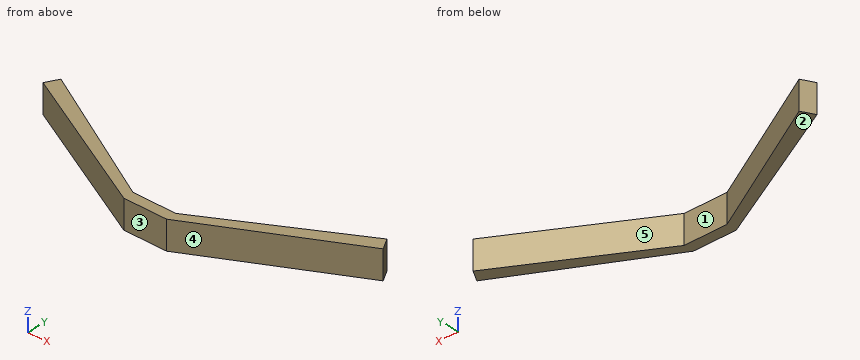
from build123d import *

# Parameters (mm, degrees)
F0_W     = 7.947458
F0_H     = 1.932221
F1_DEPTH = 5.334


with BuildPart() as f1:
    # F0 (on Top) → F1 (new body)
    with BuildSketch(Plane.XY):
        Polygon((18.552113, 1.932221), (18.552113, 0), (45.986039, 14.360375), (44.759143, 16.558673), align=None)
        Polygon((-17.014322, 14.249988), (10.604655, 0), (10.604655, 1.932221), (-15.732167, 16.558673), align=None)
        with Locations((14.578384, 0.96611)):
            Rectangle(F0_W, F0_H)
    extrude(amount=F1_DEPTH)


solid = f1.part
Read the model definition and answer for the solid it produces. Units are mm, in the model's axes. Face numbers are marked on the shaded views. A direction names the side the tool comes from. Round coordinates to 2 decimals unless told otherwise and drop trailing zeros. Write each loop counter-clockwise with the first axis right and the second up, starting at its lowest first coordinate (ties: lowest second). Pieces come first, ordered by that corner, then holes. Notation, with made-up numbers: (88.5, 75.25) - (112.5, 75.25) arc R14 ccw to (112.5, 98.25) - close; hole circle Ø1 at (9.5, 28.25). An arc over 180 degrees is marked (long way). Use a Markdown table: item, result.
(1) Straight lines are drawn through the part: line 1 along X through (y, z) = (2, 2.3); line 2 along X through (y, z) = (11.25, 2.85); line 3 along Y through (x, z) = (14, 4.15). For each, find the intervals that lie inside material, in ascending order. Write a range as [from, to].
Reported:
| item | result |
|---|---|
| line 1 | [6.73, 10.48], [18.67, 22.37] |
| line 2 | [-11.2, -6.17], [35.25, 40.04] |
| line 3 | [0, 1.93] |
(2) The part is cut by section C-C (x = 15). Write down the section's boundary in (y, z), then the cut area to 3 significant figures.
Reported:
| item | result |
|---|---|
| outline | (0, 0) - (1.93, 0) - (1.93, 5.33) - (0, 5.33) - close |
| area | 10.3 mm2 |
(3) The part is cut by section A-A (y = 3). Write down the section's boundary in (x, z).
Reported:
| item | result |
|---|---|
| outline | (4.79, 0) - (8.68, 0) - (8.68, 5.33) - (4.79, 5.33) - close; (20.47, 0) - (24.28, 0) - (24.28, 5.33) - (20.47, 5.33) - close |
(4) The part is cut by section D-D (y = 13). Write down the section's boundary in (x, z), then the cut area to 3 significant figures.
Reported:
| item | result |
|---|---|
| outline | (-14.59, 0) - (-9.32, 0) - (-9.32, 5.33) - (-14.59, 5.33) - close; (38.38, 0) - (43.39, 0) - (43.39, 5.33) - (38.38, 5.33) - close |
| area | 54.8 mm2 |
(5) Each of these flat-tipped pins is pushed along its axis until it touches: pin 1 Ø2.5 at (x, z) = (13.5, 3) entering from +Y; pin 2 Ø2 at (x, y) = (-6, 6) entering from -Z; pin 3 Ø6 at (x, y) = (27.5, 3) entering from -Z; pin 4 Ø1.5 at (y, z) = (10.5, 3.5) entering from -X. Where does it stop, or does it pass through?
Reported:
| item | result |
|---|---|
| pin 1 | y = 1.93 |
| pin 2 | through |
| pin 3 | z = 0 |
| pin 4 | x = -11.2 |
(6) The part is cut by section B-B (z = 0.6). Write down the section's boundary in (x, y).
Reported:
| item | result |
|---|---|
| outline | (-17.01, 14.25) - (10.6, 0) - (18.55, 0) - (45.99, 14.36) - (44.76, 16.56) - (18.55, 1.93) - (10.6, 1.93) - (-15.73, 16.56) - close |
(7) The mould has two halves that part along X. Classify the marked faces 3, 4 and 5: released by +X, released by -X, zero draft, split by the parting line, or undercut.
Reported:
| item | result |
|---|---|
| face 3 | zero draft |
| face 4 | released by +X |
| face 5 | undercut |
(8) Which of the six approach directions +Z, -Z, +X, -X, +Y, -Y give full straight-line access (tool end or side, diameter ignored) to the marked faces 1 and 2?
Reported:
| item | result |
|---|---|
| face 1 | +Z, -Z, +Y |
| face 2 | -Z, +X, -X, +Y, -Y |
